Geometry check sheet. Reference: the model listing, model coordinates, mm. A direction names the side the tool comes from. Round coordinates to 2 decimals unless told otherwise and drop trailing zeros. Loops run counter-clockwise (first coordinate to the right, second up) from the corner with the lowest first, then second, coordinate; pieces in that order, holes last. Notation, with made-up numbers: (6, -38.75) -> (63, -38.75) arc R7 cw to (63, -30.75) -> close; hole circle Ø10 at (47, 32.25). An arc over 180 degrees is marked (long way). Use one line per item in the form item = value.
from build123d import *

# Parameters (mm, degrees)
SKETCH1_R           = 1.6
BOSS_EXTRUDE1_DEPTH = 6
FILLET1_R           = 3
CUT_EXTRUDE1_REACH  = 124.34
SKETCH2_R           = 1.3


with BuildPart() as part:
    # Sketch1 → Boss-Extrude1 (new body)
    with BuildSketch(Plane(origin=(0, 0, 0), x_dir=(0, 0, -1), z_dir=(1, 0, 0))):
        Polygon((-65, 0), (-45, 0), (-45, 6), (55, 6), (55, 0), (75, 0), (75, 6), (91.752837084, 56.286625106), (71.728155707, 80.151111078), (-71.728155707, 80.151111078), (-92.232725383, 55.714716502), (-65, 6), align=None)
        with Locations((-85, 55)):
            Circle(SKETCH1_R, mode=Mode.SUBTRACT)
        with Locations((85, 55)):
            Circle(SKETCH1_R, mode=Mode.SUBTRACT)
        Polygon((-82.116733572, 49.736451418), (-45.025455014, 71.151111078), (-10.874545111, 12), (-61.445461749, 12), align=None, mode=Mode.SUBTRACT)
        Polygon((-39.829302592, 74.151111078), (39.829302592, 74.151111078), (3.94634188, 12), (-3.94634188, 12), align=None, mode=Mode.SUBTRACT)
        Polygon((45.025455014, 71.151111078), (83.06422235, 49.189418517), (70.674680035, 12), (10.874545111, 12), align=None, mode=Mode.SUBTRACT)
        with BuildLine():
            ThreePointArc((-61.963724259, 68.3), (-64.623217813, 72.098150418), (-67.901849582, 75.376782187))
            ThreePointArc((-67.901849582, 75.376782187), (-70.155980867, 75.179571253), (-69.958769933, 72.925439969))
            ThreePointArc((-69.958769933, 72.925439969), (-67.074560031, 70.041230067), (-64.735005551, 66.7))
            ThreePointArc((-64.735005551, 66.7), (-62.549364905, 66.114359354), (-61.963724259, 68.3))
        make_face(mode=Mode.SUBTRACT)
        with BuildLine():
            ThreePointArc((67.901849582, 75.376782187), (64.623217813, 72.098150418), (61.963724259, 68.3))
            ThreePointArc((61.963724259, 68.3), (62.549364905, 66.114359354), (64.735005551, 66.7))
            ThreePointArc((64.735005551, 66.7), (67.074560031, 70.041230067), (69.958769933, 72.925439969))
            ThreePointArc((69.958769933, 72.925439969), (70.155980867, 75.179571253), (67.901849582, 75.376782187))
        make_face(mode=Mode.SUBTRACT)
    extrude(amount=BOSS_EXTRUDE1_DEPTH)

    # Fillet1
    fillet1_edges = [part.edges().sort_by_distance(p)[0] for p in [
        (3, 49.736451418, 82.116733572),
        (3, 12, 61.445461749),
        (3, 12, 10.874545111),
        (3, 71.151111078, 45.025455014),
        (3, 74.151111078, 39.829302592),
        (3, 12, 3.94634188),
        (3, 12, -3.94634188),
        (3, 74.151111078, -39.829302592),
        (3, 71.151111078, -45.025455014),
        (3, 12, -10.874545111),
        (3, 12, -70.674680035),
        (3, 49.189418517, -83.06422235),
    ]]
    fillet(fillet1_edges, radius=FILLET1_R)

    # Sketch2 → Cut-Extrude1 (cut, up to next)
    with BuildSketch(Plane.XZ, mode=Mode.PRIVATE) as cut_extrude1_sk1:
        with Locations(Location((3, 55, 0), (0, 0, 270))):
            Circle(SKETCH2_R)
    cut_extrude1_tool1 = extrude(cut_extrude1_sk1.sketch, amount=-CUT_EXTRUDE1_REACH, mode=Mode.PRIVATE) & part.part
    # Sketch2 → Cut-Extrude1 (cut, up to next)
    with BuildSketch(Plane.XZ, mode=Mode.PRIVATE) as cut_extrude1_sk2:
        with Locations(Location((3, -65, 0), (0, 0, 270))):
            Circle(SKETCH2_R)
    cut_extrude1_tool2 = extrude(cut_extrude1_sk2.sketch, amount=-CUT_EXTRUDE1_REACH, mode=Mode.PRIVATE) & part.part
    add(cut_extrude1_tool1.solids().sort_by_distance((3, 0, 55))[0], mode=Mode.SUBTRACT)
    add(cut_extrude1_tool2.solids().sort_by_distance((3, 0, -65))[0], mode=Mode.SUBTRACT)


solid = part.part
1. Section check A-A (z = -50). Record the boundary of the cut face in (x, y), then the cut area to 3 significant figures.
Return value:
outline = (0, 6) -> (6, 6) -> (6, 12) -> (0, 12) -> close; (0, 68.28) -> (6, 68.28) -> (6, 80.15) -> (0, 80.15) -> close
area = 107 mm2
2. Section check B-B (y = 28.5). Record the boundary of the cut face in (x, z).
Return value:
outline = (0, -82.5) -> (6, -82.5) -> (6, -76.17) -> (0, -76.17) -> close; (0, -20.4) -> (6, -20.4) -> (6, -13.47) -> (0, -13.47) -> close; (0, 13.47) -> (6, 13.47) -> (6, 20.4) -> (0, 20.4) -> close; (0, 70.48) -> (6, 70.48) -> (6, 77.33) -> (0, 77.33) -> close
3. Tool access check on faces 4 (the flat face through (3, 6, -4)), 5 (the flat face through (0, 34, -20)), 6 (the cylindrical face through (3.042, 13.462, 13.495)). Record the directions out of +Z, -Z, +X, -X, +Y, -Y that give a thin tool (end or side, any length) a straight path to the whole face; none if there is none.
Return value:
face_4 = +X, -X, -Y
face_5 = +Z, -Z, -X, +Y, -Y
face_6 = +X, -X
4. Section check D-D (z = 50.5). Record the boundary of the cut face in (x, y), then the cut area to 3 significant figures.
Return value:
outline = (0, 0) -> (6, 0) -> (6, 12) -> (0, 12) -> close; (0, 67.99) -> (6, 67.99) -> (6, 80.15) -> (0, 80.15) -> close
area = 145 mm2
5. Mould release check, pull along Z, two halves, no side actions. Record for faces 1 (the flat face through (1, 0, -65)), 2 (the cylindrical face through (2.96, 55.07, -83.4)), 3 (the flat face through (2.96, 68.1, 81.84)): released by +Z, released by -Z, zero draft, split by the parting line, or undercut.
Return value:
face_1 = zero draft
face_2 = undercut
face_3 = released by +Z
6. Section check C-C (z = 23). Record the boundary of the cut face in (x, y).
Return value:
outline = (0, 6) -> (6, 6) -> (6, 12) -> (0, 12) -> close; (0, 33) -> (6, 33) -> (6, 45) -> (0, 45) -> close; (0, 74.15) -> (6, 74.15) -> (6, 80.15) -> (0, 80.15) -> close
7. Material ranges on line 1 along X through (y, z) = (6.25, -65); line 2 along Y through (x, z) = (2.3, -22); line 3 along Y through (x, z) = (3.15, -46), recorded low to high.
Return value:
line_1 = 0 to 1.7, 4.3 to 6
line_2 = 6 to 12, 31.27 to 43.27, 74.15 to 80.15
line_3 = 6 to 12, 70.05 to 80.15
8. Gauge pin test, flat ends, axial feed: pin 1 (3.5 mm diameter, centred on x = 3, z = 55, fed in from -Y); pin 2 (3 mm diameter, centred on x = 1.5, z = 12, fed in from -Y); pin 3 (3 mm diameter, centred on x = 2, y = 4, fed in from -Z); pin 4 (2 mm diameter, centred on x = 5, y = 63.5, fed in from -Z). Record the tip position at first contact, or that the pin passes through.
Return value:
pin_1 = 0
pin_2 = 6
pin_3 = -75
pin_4 = -86.54
